Autodesk Inventor part; units mm, degrees
ref_plane "YZ Plane" through (0, 0, 0) normal (1, 0, 0) x (0, 1, 0)
ref_plane "XZ Plane" through (0, 0, 0) normal (0, 1, 0) x (-1, 0, 0)
ref_plane "XY Plane" through (0, 0, 0) normal (0, 0, 1) x (1, 0, 0)
sketch "Sketch1" plane through (0, 0, 0) normal (1, 0, 0) x (0, 1, 0)
  circle A0 centre (0, 0) radius 5
  circle A1 centre (0, 0) radius 10.5
  line L0 (0, 0) -> (-20, 0)
  line L1 (-20, 0) -> (-20, -15)
  line L2 (-20, -15) -> (-20, 15)
  line L3 (-20, 15) -> (0, 10.5)
  line L4 (0, -10.5) -> (-20, -15)
  dimension "d0" = 10
  dimension "d1" = 21
  dimension "d2" = 20
  dimension "d3" = 15
  dimension "d4" = 30
extrude "Extrusion1" add sketch "Sketch1" along normal blind 5
sketch "Sketch2" plane through (5, 0, 0) normal (1, 0, 0) x (0, 0, -1)
  arc A0 (10.5, 0) -> (-10.5, 0) centre (0, 0) ccw
  circle A1 centre (0, 0) radius 10.5
  line L0 (-10.5, 0) -> (-15, -20)
  line L1 (-10.5, 0) -> (-15, -20)
  line L2 (15, -20) -> (10.5, 0)
  line L3 (-15, -20) -> (15, -20)
  line L4 (15, -20) -> (10.5, 0)
  point P0 (-10.5, 0)
extrude "Extrusion2" add sketch "Sketch2" along normal blind 10 contours L2 L3 L0 A1
sketch "Sketch4" plane through (15, 0, 0) normal (1, 0, 0) x (0, 0, -1)
  circle A0 centre (0, 0) radius 5
  circle A1 centre (0, 0) radius 10.5
  line L0 (15, -20) -> (10.5, 0)
  line L1 (10.5, 0) -> (15, -20)
  line L2 (-15, -20) -> (15, -20)
  line L3 (15, -20) -> (-15, -20)
  line L4 (-10.5, 0) -> (-15, -20)
  line L5 (-15, -20) -> (-10.5, 0)
extrude "Extrusion3" add sketch "Sketch4" along normal blind 5
sketch "Sketch5" plane through (0, -20, -15) normal (0, -1, 0) x (1, 0, 0)
  line L0 (20, 4.5) -> (20, 25.5)
  line L1 (20, 15) -> (0, 15)
  circle A0 centre (10, 15) radius 5
  dimension "d11" = 10
extrude "Extrusion4" add sketch "Sketch5" along normal blind 30
fillet "Fillet1" radius 5 6 edges at (20, -10, 12.75) (20, -10, -12.75) (20, 10.5, 0) (0, 10.5, 0) (0, -10, -12.75) (0, -10, 12.75)
properties part number "wrist"
Geometry check sheet. Reference: the model listing, model coordinates, mm. A direction names the side the tool comes from. Round coordinates to 2 decimals unless told otherwise and drop trailing zeros. Loops run counter-clockwise (first coordinate to the right, second up) from the corner with the lowest first, then second, coordinate; pieces in that order, holes last. Notation, with made-up numbers: M 41.25,1 L 63.25,1 A22 ccw 63.25,15 Z; hole C 45,-8 d4. An arc over 180 degrees is marked long. Return JSON: item names as keys, results as strings. Group by question number.
(1) Set-up check for faces 1 (the face through (14.77, -34.79, -1.5)), 2 (the face through (5, 5, -2)), 3 (the face through (9.93, -10.14, -12.78)): record each of +Z, -Z, +X, -X, +Y, -Y from which the full face is reachable in a straight line by a thin tool's end or side.
(2) Section check D-D, the plane y = -38.5. Enter the section's corners in (x, z).
(3) Go/stop test with flat-tipped pins: pin 1 (1 mm diameter, centred on x = 3.5, z = 6.5, fed in from -Y); pin 2 (10 mm diameter, centred on x = 15.5, y = -35.5, fed in from -Z); pin 3 (5 mm diameter, centred on y = -22, z = -12, fed in from +X). Record where each tip stops, or that it passes through.
(4) Mould release check, pull along Z, two halves, no side actions. Record for faces 4 (the face through (17.46, 4.88, 1.08)), 5 (the face through (14.3, -20, -3.1)), 6 (the face through (18.574, -9.87, -11.18)): pulls with the +Z half, pulls with the -Z half, needs draft (parallel to the pull), parting line crosses it, or undercut.
(5) Section check C-C, the plane x = 15.75. Enter the section's corners in (y, z).
(6) Section check A-A, the plane z = 0. Give the number of separate pieces and of enclosed holes in the cut face, and give its area (3 significant figures).
(7) Section check B-B, the plane x = 10. Enter the section's corners in (y, z).
(8) Scan lines: line 1 along Y through (x, z) = (1.95, 0); line 2 along Y through (x, z) = (3, 0); line 3 along Z through (x, y) = (15.5, -0.5). Record each from-to range of solid material in increasing order. Write a range as [from, to].
Data:
{
 "1": {"face 1": "-Y", "face 2": "+Y", "face 3": "-Z, +X, -X, +Y"},
 "2": {"outline": "C 10,0 d10"},
 "3": {"pin 1": "y = -20", "pin 2": "z = -4.97", "pin 3": "x = 19.96"},
 "4": {"face 4": "undercut", "face 5": "needs draft", "face 6": "pulls with the -Z half"},
 "5": {"outline": "M -20,-14.94 L -0.01,-10.44 A10.44 ccw -0.01,10.44 L -20,14.94 Z; hole C 0,0 d10"},
 "6": {"separate pieces": "3", "enclosed holes": "0", "area": "589 mm²"},
 "7": {"outline": "M -50,-5 L -20,-5 L -20,-15 L 0,-10.5 A10.5 cw 0,10.5 L -20,15 L -20,5 L -50,5 Z"},
 "8": {"line 1": "[-20, -5], [5, 9.46]", "line 2": "[-20, -5], [5, 10.08]", "line 3": "[-10.59, -4.97], [4.97, 10.59]"}
}
